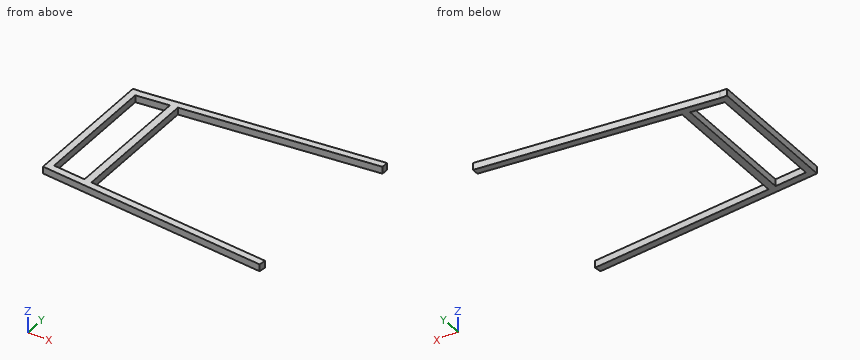
from build123d import *

# Parameters (mm, degrees)
F1_DEPTH = 30


with BuildPart() as f1:
    # F0 (on Top) → F1 (new body)
    with BuildSketch(Plane.XY):
        Polygon((-45.581206, 304.954057), (-75.581206, 304.954057), (-75.581206, -295.045943), (-45.581206, -295.045943), (-45.581206, -267.712643), (-45.581206, 273.296505), align=None)
        Polygon((-45.581206, -295.045943), (-75.581206, -295.045943), (924.418794, -404.579163), (927.732864, -374.322866), (126.900651, -286.605136), (94.68448, -283.076395), (-45.581206, -267.712643), align=None)
        Polygon((126.900651, 289.434935), (94.68448, 286.420598), (94.68448, -283.076395), (126.900651, -286.605136), align=None)
        Polygon((955.307603, 396.427751), (-45.581206, 304.954057), (-45.581206, 273.296505), (94.68448, 286.420598), (126.900651, 289.434935), (955.307603, 366.945624), align=None)
    extrude(amount=F1_DEPTH)


solid = f1.part
Geometry: final body of the model. Coordinates: model frame, mm. Give positions to 0.01 mm unless a question says otherwise; leave off trailing zeros. Write each loop counter-clockwise with the first axis right and the second up, starting at its lowest first coordinate (ties: lowest second). Pieces come first, ordered by that corner, then holes. Notation, with made-up numbers: M 4.25,47 L 9.25,47 A16 cw 9.25,58 Z; hole C 59,-39.75 d3. An arc over 180 degrees is marked long. Answer in a Markdown table with one row per item. Add a question column.
(1) Section B-B on y = -28.5. Return loops of the section in (x, z), and give its area (3 significant figures).
(2) Section A-A on z = 12.5. Return loops of the section in (x, y), and give its area (4 significant figures).
(3) Section C-C on x = 9.5. Return loops of the section in (y, z).
(4) Ray query, line 1 (X direction, y = 133, z = 14.75); line 2 (Y direction, x = 331, z = 27); line 3 (Y direction, x = 413, z = 14.5). Return the intervals inside material, ascending.
(5) First-contact query: pin 1 (15 mm diameter, centred on y = -36.5, z = 21.5, fed in from +X); pin 2 (4 mm diameter, centred on x = 177.5, z = 25.5, fed in from +Y); pin 3 (5 mm diameter, centred on x = 117.5, z = 3.5, fed in from +Y). Flat tips, straight axial feed; report the tip coordinate or a pass-through.
Result set:
| question | item | result |
|---|---|---|
| 1 | outline | M -75.58,0 L -45.58,0 L -45.58,30 L -75.58,30 Z; M 94.68,0 L 126.9,0 L 126.9,30 L 94.68,30 Z |
| 1 | area | 1,870 mm^2 |
| 2 | outline | M -75.58,-295.05 L 924.42,-404.58 L 927.73,-374.32 L 126.9,-286.61 L 126.9,289.43 L 955.31,366.95 L 955.31,396.43 L -45.58,304.95 L -75.58,304.95 Z; hole M -45.58,-267.71 L 94.68,-283.08 L 94.68,286.42 L -45.58,273.3 Z |
| 2 | area | 96,850 mm^2 |
| 3 | outline | M -304.37,0 L -273.75,0 L -273.75,30 L -304.37,30 Z; M 278.45,0 L 309.99,0 L 309.99,30 L 278.45,30 Z |
| 4 | line 1 | x = -75.58 to -45.58, 94.68 to 126.9 |
| 4 | line 2 | y = -339.58 to -308.96, 308.53 to 339.37 |
| 4 | line 3 | y = -348.56 to -317.94, 316.2 to 346.86 |
| 5 | pin 1 | stops at x = 126.9 |
| 5 | pin 2 | stops at y = 325.52 |
| 5 | pin 3 | stops at y = 320.09 |
